Work out the finished part from the listing and answer in its coordinate system (mm). A direction names the side the tool comes from. Coordinates: 2 decimals unless noted, no trailing zeros. Order: outer loops, then holes, each group sorted by start corner. A loop starts at its lowest first (then second) coordinate and runs counter-clockwise, first axis right, second up. Notation, with made-up numbers: (37, 5) -> (46, 5) arc R24 cw to (46, 19) -> close; hole circle Ø7 at (13, 15.5). An arc over 180 degrees is marked (long way). Write item = value, one per line. Start each with the question number.
Q1. A flat-ended cylindrical pin translates along its axis: pin 1 (3 mm diameter, centred on x = 10.5, y = -24.5, fed in from +Z). Find the tip coordinate at first contact, or state that the pin passes through.
Q2. The part is cut by section C-C, the plane y = -22.4. Determine the outline of the cut face in (x, z), plus the area to 3 significant figures.
Q3. The part is cut by section A-A, the plane x = 0. Determine the outline of the cut face in (y, z).
Q4. For a pull along X with two mould halves and no side action, classify faces 1 (the cylindrical face through (25.005, -2.18, 10.768)), 2 (the flat face through (40, -3, 6)), 3 (the flat face through (-40, -2, 6)) as +X half, -X half, draft (parallel to the pull), parting line (faces both ways), or undercut.
Q5. The part is cut by section B-B, the plane x = 23.57. Determine the outline of the cut face in (y, z).
Q6. Straight lines are drawn through the part: L1, parallel to X at y = 23.5, z = 5.75; L2, parallel to Y at x = 30, z = 10; L3, parallel to X at y = 23, z = 11. For each, find the intervals that lie inside material, in ascending order. Write a range as from..to.
Q7. Which of the six approach directions +Z, -Z, +X, -X, +Y, -Y give full straight-line access (tool end or side, diameter ignored) to faces 4 (the flat face through (1.89, 5.45, 5)), 5 (the cylindrical face through (-23.11, 21.59, 5.92)), 6 (the flat face through (12, -25, 9.5))?
Q8. The part is cut by section D-D, the plane z = 3.25. Count the separate pieces of the cut face and the enclosed holes in it, plus the area to 3 significant figures.
```python
from build123d import *

# Parameters (mm, degrees)
BOSS_EXTRUDE1_DEPTH                                 = 12
M5_TAPPED_HOLE1_D                                   = 4.2
CBORE_FOR_M5_HEX_SOCKET_HEAD_CAP_SCREW1_D           = 5.3
CBORE_FOR_M5_HEX_SOCKET_HEAD_CAP_SCREW1_CBORE_D     = 10
CBORE_FOR_M5_HEX_SOCKET_HEAD_CAP_SCREW1_CBORE_DEPTH = 2.5
SKETCH8_R                                           = 5.6
CUT_EXTRUDE1_DEPTH                                  = 12
SKETCH9_R                                           = 8
CUT_EXTRUDE2_DEPTH                                  = 5


with BuildPart() as part:
    # Sketch3 → Boss-Extrude1 (new body)
    with BuildSketch(Plane.XY):
        Polygon((-40, -32.4), (40, -32.4), (40, 27.54), (35, 32.54), (-35, 32.54), (-40, 27.54), align=None)
    extrude(amount=BOSS_EXTRUDE1_DEPTH)

    # M5 Tapped Hole1 (through all)
    with Locations(Plane.XY.offset(12)):
        with Locations((-23.57, -23.5), (-23.57, 23.64), (23.57, 23.64), (23.57, -23.5)):
            Hole(M5_TAPPED_HOLE1_D / 2)

    # CBORE for M5 Hex Socket Head Cap Screw1 (through all)
    with Locations(Plane.XY.offset(12)):
        with Locations((-30, -2.4), (-10, -22.4), (10, -22.4), (30, -2.4)):
            CounterBoreHole(CBORE_FOR_M5_HEX_SOCKET_HEAD_CAP_SCREW1_D / 2, CBORE_FOR_M5_HEX_SOCKET_HEAD_CAP_SCREW1_CBORE_D / 2, CBORE_FOR_M5_HEX_SOCKET_HEAD_CAP_SCREW1_CBORE_DEPTH)

    # Sketch8 → Cut-Extrude1 (cut)
    with BuildSketch(Plane.XY.offset(12)):
        Circle(SKETCH8_R)
    extrude(amount=-CUT_EXTRUDE1_DEPTH, mode=Mode.SUBTRACT)

    # Sketch9 → Cut-Extrude2 (cut)
    with BuildSketch(Plane(origin=(0, 0, 0), x_dir=(-1, 0, 0), z_dir=(0, 0, -1))):
        Circle(SKETCH9_R)
    extrude(amount=-CUT_EXTRUDE2_DEPTH, mode=Mode.SUBTRACT)


solid = part.part
```
Model answer:
q1.pin_1 = 9.5
q2.outline = (-40, 0) -> (-25.36, 0) -> (-25.36, 12) -> (-40, 12) -> close; (-21.78, 0) -> (-12.65, 0) -> (-12.65, 9.5) -> (-15, 9.5) -> (-15, 12) -> (-21.78, 12) -> close; (-7.35, 0) -> (7.35, 0) -> (7.35, 9.5) -> (5, 9.5) -> (5, 12) -> (-5, 12) -> (-5, 9.5) -> (-7.35, 9.5) -> close; (12.65, 0) -> (21.78, 0) -> (21.78, 12) -> (15, 12) -> (15, 9.5) -> (12.65, 9.5) -> close; (25.36, 0) -> (40, 0) -> (40, 12) -> (25.36, 12) -> close
q2.area = 723 mm2
q3.outline = (-32.4, 0) -> (-8, 0) -> (-8, 5) -> (-5.6, 5) -> (-5.6, 12) -> (-32.4, 12) -> close; (5.6, 5) -> (8, 5) -> (8, 0) -> (32.54, 0) -> (32.54, 12) -> (5.6, 12) -> close
q4.face_1 = undercut
q4.face_2 = +X half
q4.face_3 = -X half
q5.outline = (-32.4, 0) -> (-25.6, 0) -> (-25.6, 12) -> (-32.4, 12) -> close; (-21.4, 0) -> (21.54, 0) -> (21.54, 12) -> (-21.4, 12) -> close; (25.74, 0) -> (32.54, 0) -> (32.54, 12) -> (25.74, 12) -> close
q6.L1 = -40..-25.67, -21.47..21.47, 25.67..40
q6.L2 = -32.4..-7.4, 2.6..32.54
q6.L3 = -40..-25.57, -21.57..21.57, 25.57..40
q7.face_4 = -Z
q7.face_5 = +Z, -Z
q7.face_6 = +Z
q8.separate_pieces = 1
q8.enclosed_holes = 9
q8.area = 4,830 mm2
